```python
from build123d import *

# Parameters (mm, degrees)
Y_KSEKLIK_EKSTR_ZYON1_DEPTH = 5
IZIM2_W                     = 15
IZIM2_H                     = 5
KES_EKSTR_ZYON1_DEPTH       = 10
IZIM4_R                     = 1
Y_KSEKLIK_EKSTR_ZYON2_DEPTH = 2.5
IZIM5_R                     = 1.5
KES_EKSTR_ZYON2_DEPTH       = 5


with BuildPart() as part:
    # Çizim1 → Yükseklik-Ekstrüzyon1 (new body, symmetric)
    with BuildSketch(Plane.XY):
        Polygon((-29.798797212, 38.403805497), (-4.798797212, 38.403805497), (-4.798797212, 40.403805497), (-31.798797212, 40.403805497), (-31.798797212, 38.403805497), align=None)
    extrude(amount=Y_KSEKLIK_EKSTR_ZYON1_DEPTH, both=True)

    # Çizim2 → Kes-Ekstrüzyon1 (cut)
    with BuildSketch(Plane(origin=(0, 40.403805497, 0), x_dir=(1, 0, 0), z_dir=(0, 1, 0))):
        with Locations((-31.798797212, 0)):
            Rectangle(IZIM2_W, IZIM2_H)
    extrude(amount=-KES_EKSTR_ZYON1_DEPTH, mode=Mode.SUBTRACT)

    # Çizim4 → Yükseklik-Ekstrüzyon2 (add, symmetric)
    with BuildSketch(Plane.XY):
        with Locations((-28.798797212, 39.403805497)):
            Circle(IZIM4_R)
    extrude(amount=Y_KSEKLIK_EKSTR_ZYON2_DEPTH, both=True)

    # Çizim5 → Kes-Ekstrüzyon2 (cut)
    with BuildSketch(Plane(origin=(0, 40.403805497, 0), x_dir=(1, 0, 0), z_dir=(0, 1, 0))):
        with Locations((-14.798797212, 0)):
            Circle(IZIM5_R)
    extrude(amount=-KES_EKSTR_ZYON2_DEPTH, mode=Mode.SUBTRACT)


solid = part.part
```
Input: part model. Units: mm. Frame: model coordinates. A direction names the side the tool comes from. Round coordinates to 2 decimals unless told otherwise and drop trailing zeros. Loops run counter-clockwise (first coordinate to the right, second up) from the corner with the lowest first, then second, coordinate; pieces in that order, holes last.
1) Material intervals for line 1 (Z direction, x = -26.75, y = 38.65); line 2 (X direction, y = 40.05, z = 0); line 3 (X direction, y = 39.15, z = 0), sorted ascending.
Ans:
line 1: z = -5 to -2.5, 2.5 to 5
line 2: x = -29.56 to -28.04, -24.3 to -16.3, -13.3 to -4.8
line 3: x = -29.77 to -27.83, -24.3 to -16.3, -13.3 to -4.8
2) Section query A-A on x = -26. Return the cut outline in (y, z), plus the area to 3 significant figures.
Ans:
outline: (38.4, -5) - (40.4, -5) - (40.4, -2.5) - (38.4, -2.5) - close; (38.4, 2.5) - (40.4, 2.5) - (40.4, 5) - (38.4, 5) - close
area: 10.0 mm2
3) Section query C-C on y = 39.7. Return the cut outline in (x, z).
Ans:
outline: (-31.8, -5) - (-4.8, -5) - (-4.8, 5) - (-31.8, 5) - (-31.8, 2.5) - (-29.75, 2.5) - (-29.75, -2.5) - (-31.8, -2.5) - close; hole (-27.84, -2.5) - (-24.3, -2.5) - (-24.3, 2.5) - (-27.84, 2.5) - close; hole circle Ø3 at (-14.8, 0)
4) Set-up query: faces 1 (the flat face through (-31.799, 39, -4)), 2 (the cylindrical face through (-28.337, 38.517, 0.035)). Return all of +Z, -Z, +X, -X, +Y, -Y with unobstructed straight access to the full face (end or side cutting, diameter ignored); none if empty.
Ans:
face 1: +Z, -Z, -X, +Y, -Y
face 2: none
5) Section query D-D on z = 2. Return the cut outline in (x, y), plus the area to 3 significant figures.
Ans:
outline: circle Ø2 at (-28.8, 39.4); (-24.3, 38.4) - (-4.8, 38.4) - (-4.8, 40.4) - (-24.3, 40.4) - close
area: 42.1 mm2
6) Section query B-B on z = 0. Return the cut outline in (x, y).
Ans:
outline: circle Ø2 at (-28.8, 39.4); (-24.3, 38.4) - (-16.3, 38.4) - (-16.3, 40.4) - (-24.3, 40.4) - close; (-13.3, 38.4) - (-4.8, 38.4) - (-4.8, 40.4) - (-13.3, 40.4) - close
7) Pin query (flat end, axial travel): pin 1 (5 mm diameter, centred on x = -14.8, z = 0, fed in from -Y). Return the tip coordinate at first contact, or that it passes through.
Ans:
pin 1: stops at y = 38.4
8) Pull-direction query (Z, two-part tool) for faces 3 (the flat face through (-4.799, 39, 0)), 4 (the flat face through (-24.299, 39, 0)), 5 (the flat face through (-18, 39, 5)); classes: released by +Z, released by -Z, zero draft, split by the parting line, or undercut.
Ans:
face 3: zero draft
face 4: undercut
face 5: released by +Z
